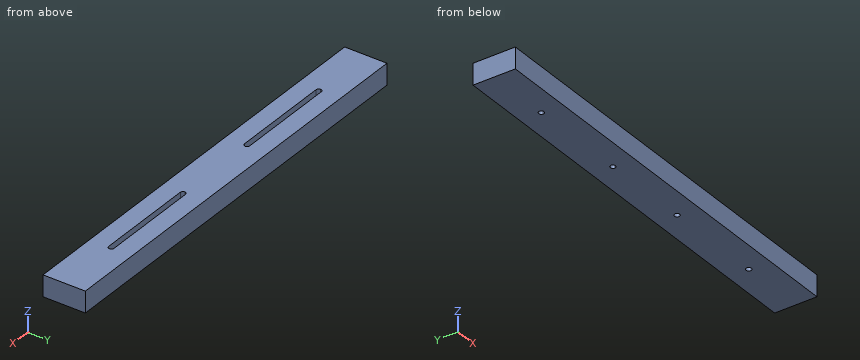
```python
from build123d import *

# Parameters (mm, degrees)
F0_W     = 40
F0_H     = 4
F1_DEPTH = 2
F2_W     = 10
F2_H     = 0.5
F3_DEPTH = 1
F4_R     = 0.25
F5_DEPTH = 25
F6_R     = 0.24999


# Not quite as in the source:
# - a fillet or chamfer is up to 0.001 mm smaller than in the source, because OpenCascade refuses the exact size


with BuildPart() as f1:
    # F0 (on Top) → F1 (new body)
    with BuildSketch(Plane.XY):
        Rectangle(F0_W, F0_H)
    extrude(amount=F1_DEPTH)

    # F2 (on face) → F3 (cut)
    with BuildSketch(Plane.XY.offset(2)):
        with Locations((-9, 0)):
            Rectangle(F2_W, F2_H)
        with Locations((9, 0)):
            Rectangle(F2_W, F2_H)
    extrude(amount=-F3_DEPTH, mode=Mode.SUBTRACT)

    # F4 (on face) → F5 (cut)
    with BuildSketch(Plane.XY.offset(1)):
        with BuildLine():
            ThreePointArc((-13.75, -0.25), (-13.5732233047, -0.1767766953), (-13.5, 0))
            ThreePointArc((-13.5, 0), (-13.5732233047, 0.1767766953), (-13.75, 0.25))
            ThreePointArc((-13.75, 0.25), (-13.9267766953, 0.1767766953), (-14, 0))
            ThreePointArc((-14, 0), (-13.9267766953, -0.1767766953), (-13.75, -0.25))
        make_face()
        with BuildLine():
            ThreePointArc((-4, 0), (-4.0732233047, 0.1767766953), (-4.25, 0.25))
            ThreePointArc((-4.25, 0.25), (-4.5, 0), (-4.25, -0.25))
            ThreePointArc((-4.25, -0.25), (-4.0732233047, -0.1767766953), (-4, 0))
        make_face()
        with Locations((13.75, 0)):
            Circle(F4_R)
        with Locations((4.25, 0)):
            Circle(F4_R)
    extrude(amount=-F5_DEPTH, mode=Mode.SUBTRACT)

    # F6 (radius 0.25 in the source; OpenCascade refuses exactly that, so slightly less here)
    f6_edges = [f1.edges().sort_by_distance(p)[0] for p in [
        (14, 0.25, 1.5),
        (14, -0.25, 1.5),
        (4, -0.25, 1.5),
        (4, 0.25, 1.5),
        (-14, 0.25, 1.5),
        (-14, -0.25, 1.5),
        (-4, 0.25, 1.5),
        (-4, -0.25, 1.5),
    ]]
    fillet(f6_edges, radius=F6_R)


solid = f1.part
```
Can you work these out from the model? Positions are in its coordinate system, mm. Coordinates: 2 decimals unless noted, no trailing zeros. Order: outer loops, then holes, each group sorted by start corner. A loop starts at its lowest first (then second) coordinate and runs counter-clockwise, first axis right, second up.
1. I need wall thicknesses on line 1 (Y direction, x = 13.75, z = 0.45); line 2 (Z direction, x = 9, y = -0.2). Which ranges of each line are inside material? Lowest first, please.
2. If we section it at B-B (x = 12.5): Please give me the cut outline in (y, z).
3. If we section it at A-A (z = 1.55): Give the number of separate pieces and of enclosed holes in the cut face, then the cut area to 3 significant figures.
Entries:
1. line 1: y = -2 to -0.25, 0.25 to 2
1. line 2: z = 0 to 1
2. outline: (-2, 0) - (2, 0) - (2, 2) - (0.25, 2) - (0.25, 1) - (-0.25, 1) - (-0.25, 2) - (-2, 2) - close
3. separate pieces: 1
3. enclosed holes: 2
3. area: 150 mm2
